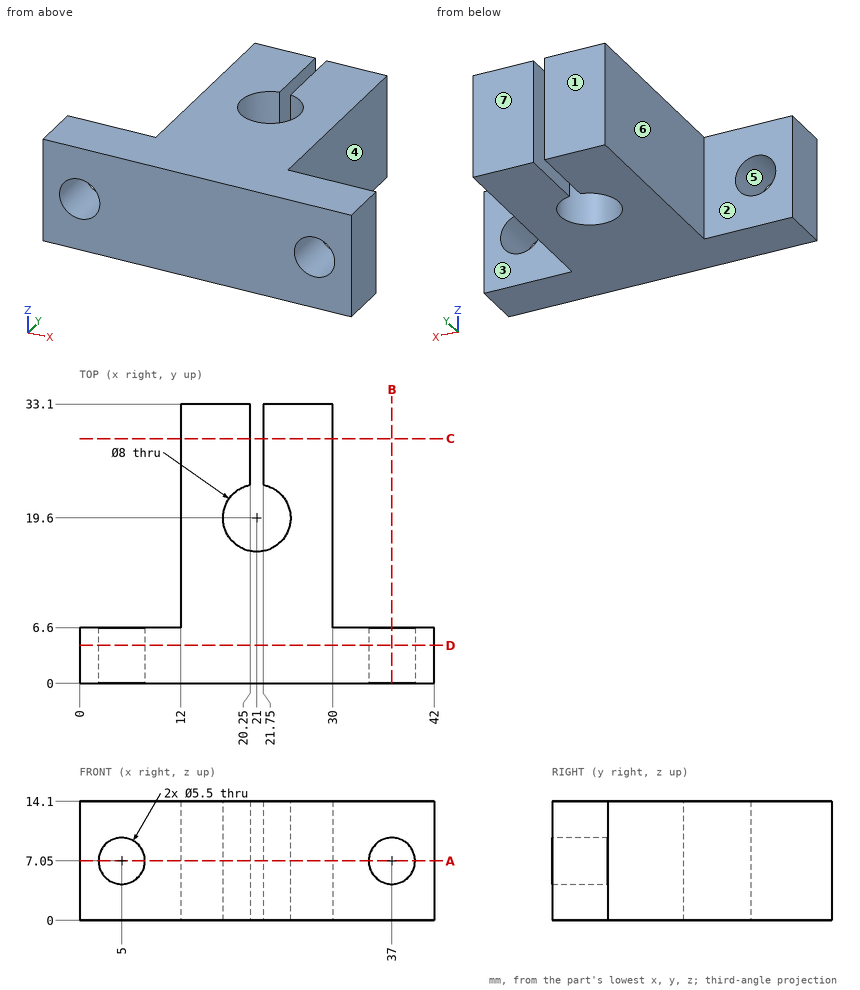
Can you work these out from the drawing? Everything is in mm from the part's minimum corner. A direction names the side the tool comes from. Round coordinates to 2 decimals unless told otherwise and drop trailing zeros. Write each loop counter-clockwise with the first axis right and the second up, starting at its lowest first coordinate (ties: lowest second). Pieces come first, ordered by that corner, then holes. Notation, with made-up numbers: (-11.75, 0.25) - (6.25, 0.25) arc R22 cw to (6.25, 25.25) - close; hole circle Ø5 at (87, 28). An arc over 180 degrees is marked (long way). Put each result on its own line as item: value. Start each with the question number.
(1) I want a section at D-D, the plane y = 4.5. Please give me the cut outline in (x, z), plus the area to 3 significant figures.
(2) I want a section at A-A, the plane z = 7.05. Please give me the cut outline in (x, y), plus the area to 3 significant figures.
(3) I need wall thicknesses on probe 1 along X at (y, z) = (2.5, 7.05); probe 2 along X at (y, z) = (19.6, 4.5); probe 3 along X at (y, z) = (24.5, 5.5). Which ranges of each line are inside material? Lowest first, please.
(4) Thinking about a two-plate mould opening in X: for the marked faces 4, 5, 6 and 7, which applies, released by +X, released by -X, zero draft, split by the parting line, or undercut?
(5) I want a section at C-C, the plane y = 29. Please give me the cut outline in (x, z), plus the area to 3 significant figures.
(6) For the marked faces 1, 2 and 3, which set-ups out of +Z, -Z, +X, -X, +Y, -Y let a thin tool reach every point of the face, with its end or its side?
(7) Will these pins go through, and if not, where does the flat tip stop? pin 1 (4 mm diameter, centred on y = 24, z = 10, fed in from -X); pin 2 (3.5 mm diameter, centred on x = 5.5, z = 8, fed in from +Y); pin 3 (6 mm diameter, centred on y = 11, z = 11, fed in from +X).
(8) I want a section at B-B, the plane x = 37. Please give me the cut outline in (y, z), plus the area to 3 significant figures.
Here are the results:
1. outline: (0, 0) - (42, 0) - (42, 14.1) - (0, 14.1) - close; hole circle Ø5.5 at (5, 7.05); hole circle Ø5.5 at (37, 7.05)
1. area: 545 mm^2
2. outline: (0, 0) - (2.25, 0) - (2.25, 6.6) - (0, 6.6) - close; (7.75, 0) - (34.25, 0) - (34.25, 6.6) - (30, 6.6) - (30, 33.1) - (21.75, 33.1) - (21.75, 23.53) arc R4 cw (long way) to (20.25, 23.53) - (20.25, 33.1) - (12, 33.1) - (12, 6.6) - (7.75, 6.6) - close; (39.75, 0) - (42, 0) - (42, 6.6) - (39.75, 6.6) - close
2. area: 617 mm^2
3. probe 1: x = 0 to 2.25, 7.75 to 34.25, 39.75 to 42
3. probe 2: x = 12 to 17, 25 to 30
3. probe 3: x = 12 to 20.25, 21.75 to 30
4. face 4: released by +X
4. face 5: undercut
4. face 6: released by -X
4. face 7: zero draft
5. outline: (12, 0) - (20.25, 0) - (20.25, 14.1) - (12, 14.1) - close; (21.75, 0) - (30, 0) - (30, 14.1) - (21.75, 14.1) - close
5. area: 233 mm^2
6. face 1: +Z, -Z, +X, -X, +Y
6. face 2: +Z, -Z, -X, +Y
6. face 3: +Z, -Z, +X, +Y
7. pin 1: stops at x = 12
7. pin 2: stops at y = 6.6
7. pin 3: stops at x = 30
8. outline: (0, 0) - (6.6, 0) - (6.6, 4.3) - (0, 4.3) - close; (0, 9.8) - (6.6, 9.8) - (6.6, 14.1) - (0, 14.1) - close
8. area: 56.8 mm^2
